from build123d import *

# Parameters (mm, degrees)
F0_R     = 14.2875
F1_DEPTH = 41.148
F0_R_2   = 6.35
F2_DEPTH = 11.176
F4_DEPTH = 3.175


with BuildPart() as f1:
    # F0 (on Top) → F1 (new body)
    with BuildSketch(Plane.XY):
        with BuildLine():
            ThreePointArc((23.36292, -9.966643), (24.88552, -5.086346), (25.4, 0))
            ThreePointArc((25.4, 0), (-5.086346, 24.88552), (-23.36292, -9.966643))
            ThreePointArc((-23.36292, -9.966643), (0, -25.4), (23.36292, -9.966643))
        make_face()
        Circle(F0_R, mode=Mode.SUBTRACT)
    extrude(amount=F1_DEPTH)

    # F0 (on Top) → F2 (join)
    with BuildSketch(Plane.XY):
        with BuildLine():
            ThreePointArc((-23.36292, -9.966643), (-5.086346, 24.88552), (25.4, 0))
            ThreePointArc((25.4, 0), (24.88552, -5.086346), (23.36292, -9.966643))
            Line((23.36292, -9.966643), (46.09719, 43.325018))
            ThreePointArc((46.09719, 43.325018), (44.469982, 61.300097), (28.575, 69.85))
            Line((28.575, 69.85), (-28.575, 69.85))
            ThreePointArc((-28.575, 69.85), (-44.469982, 61.300097), (-46.09719, 43.325018))
            Line((-46.09719, 43.325018), (-23.36292, -9.966643))
        make_face()
        with Locations((-28.575, 50.8)):
            Circle(F0_R_2, mode=Mode.SUBTRACT)
        with Locations((28.575, 50.8)):
            Circle(F0_R_2, mode=Mode.SUBTRACT)
    extrude(amount=F2_DEPTH)

    # F3 (on Right) → F4 (join, symmetric)
    with BuildSketch(Plane.YZ):
        Polygon((66.675, 11.176), (25.4, 35.006132), (25.4, 11.176), align=None)
        Polygon((25.4, 11.176), (25.4, 35.006132), (22.225, 36.839219), (22.225, 11.176), align=None)
    extrude(amount=F4_DEPTH, both=True)


solid = f1.part
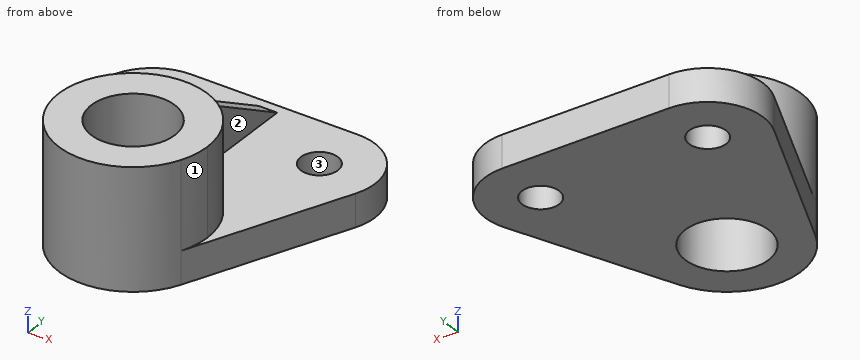
Verification items for the finished model (mm, model axes). Face numbers are marked on the shaded views. Give positions to 0.01 mm unless a question says otherwise; leave off trailing zeros. Loops run counter-clockwise (first coordinate to the right, second up) from the corner with the lowest first, then second, coordinate; pieces in that order, holes last.
1) Sectioned sample at D-D, the plane y = 49.5. Enter the section's corners in (x, z) (1 decimal).
2) Draft check along Y on the marked faces 1, 2 and 3. Enter one of: pulls with the +Y half, pulls with the -Y half, needs draft (parallel to the pull), parting line crosses it, or undercut.
3) Sectioned sample at B-B, the plane y = -8. Enter the section's corners in (x, z), then the cut area to 3 significant figures.
4) Depth check by flat-ended pin: pin 1 Ø4 at (x, y) = (-5.5, 19) entering from -Z; pin 2 Ø8 at (x, y) = (2, 57.5) entering from +Z; pin 3 Ø5 at (x, z) = (7, 7) entering from -Y; pin 4 Ø2 at (y, z) = (38.5, 16) entering from +X (3 decimals). Enter the tip coordinate at first touch or a pass-through.
5) Thickness scan on line 1 along X through (y, z) = (50, 4); line 2 along Z through (x, y) = (-36, 28.5); line 3 along Y through (x, z) = (4, 4). Record the ranges inside material, lowest first.
6) Sectioned sample at C-C, the plane x = 5.5. Enter the section's corners in (y, z).
7) Sectioned sample at A-A, the plane z = 4. Count the separate pieces of the cut face and the enclosed holes in it, then the cut area to 3 significant figures.
Answers:
1. outline: (-47.6, 0) - (-34.8, 0) - (-34.8, 11.2) - (-47.6, 11.2) - close; (-22.4, 0) - (22.4, 0) - (22.4, 11.2) - (3.2, 11.2) - (3.2, 21.1) - (-3.2, 21.1) - (-3.2, 11.2) - (-22.4, 11.2) - close; (34.8, 0) - (47.6, 0) - (47.6, 11.2) - (34.8, 11.2) - close
2. face 1: pulls with the -Y half
2. face 2: needs draft
2. face 3: undercut
3. outline: (-24.2, 0) - (-11.84, 0) - (-11.84, 41.15) - (-24.11, 41.15) - (-24.11, 11.18) - (-24.2, 11.18) - close; (11.84, 0) - (24.2, 0) - (24.2, 11.18) - (24.11, 11.18) - (24.11, 41.15) - (11.84, 41.15) - close
3. area: 1,010 mm2
4. pin 1: stops at z = 0
4. pin 2: stops at z = 18.78
4. pin 3: stops at y = -25
4. pin 4: stops at x = 3.175
5. line 1: x = -47.61 to -34.87, -22.28 to 22.28, 34.87 to 47.61
5. line 2: z = 0 to 11.18
5. line 3: y = -25.08 to -13.72, 13.72 to 69.85
6. outline: (-24.8, 0) - (-13.19, 0) - (-13.19, 41.15) - (-24.8, 41.15) - close; (13.19, 0) - (69.85, 0) - (69.85, 11.18) - (24.8, 11.18) - (24.8, 41.15) - (13.19, 41.15) - close
7. separate pieces: 1
7. enclosed holes: 3
7. area: 5,690 mm2
